```python
from build123d import *

# Parameters (mm, degrees)
SKETCH1_R           = 1.4
BOSS_EXTRUDE1_DEPTH = 2
BOSS_EXTRUDE2_START = -12.5
BOSS_EXTRUDE2_DEPTH = 10
SKETCH2_R           = 2
CUT_EXTRUDE1_DEPTH  = 40.088742751
CUT_EXTRUDE2_START  = -4
SKETCH2_3_R         = 2
CUT_EXTRUDE2_DEPTH  = 36.088742751
SKETCH4_W           = 3.030010437
SKETCH4_H           = 28.00665459
CUT_EXTRUDE3_DEPTH  = 40.088742751


# Read off the part's stored shape, not the designer's step: Boss-Extrude2
with BuildPart() as part:
    # Sketch1 → Boss-Extrude1 (new body)
    with BuildSketch(Plane.XY):
        with BuildLine():
            Line((7.5, -2.5), (7.5, 6.273123532))
            ThreePointArc((7.5, 6.273123532), (6.401650429, 8.924773961), (3.75, 10.023123532))
            Line((3.75, 10.023123532), (0, 10.023123532))
            Line((0, 10.023123532), (0, 13))
            Line((0, 13), (-29.5, 13))
            Line((-29.5, 13), (-29.5, 10.023123532))
            Line((-29.5, 10.023123532), (-33.25, 10.023123532))
            ThreePointArc((-33.25, 10.023123532), (-35.901650429, 8.924773961), (-37, 6.273123532))
            Line((-37, 6.273123532), (-37, -2.5))
            Line((-37, -2.5), (7.5, -2.5))
        make_face()
        with Locations((3.75, 6.273123532)):
            Circle(SKETCH1_R, mode=Mode.SUBTRACT)
        with Locations((-33.25, 6.273123532)):
            Circle(SKETCH1_R, mode=Mode.SUBTRACT)
    extrude(amount=BOSS_EXTRUDE1_DEPTH)

    # Boss-Extrude2 outline → Boss-Extrude2 (add)
    with BuildSketch(Plane(origin=(0, 0, 0), x_dir=(1, 0, 0), z_dir=(0, 1, 0)).offset(BOSS_EXTRUDE2_START)):
        Polygon((7.5, 44.633095244), (-37, 0.133095244), (-37, -2), (7.5, -2), align=None)
    extrude(amount=BOSS_EXTRUDE2_DEPTH)

    # Sketch2 → Cut-Extrude1 (cut, through all)
    with BuildSketch(Plane(origin=(-18.566547622, 0, -18.566547622), x_dir=(-0.7071067811865457, 0, 0.7071067811865495), z_dir=(-0.7071067811865495, 0, -0.7071067811865457))):
        with Locations((4.603838354, -7.5)):
            Circle(SKETCH2_R)
        with Locations((-15.396161646, -7.5)):
            Circle(SKETCH2_R)
    extrude(amount=-CUT_EXTRUDE1_DEPTH, mode=Mode.SUBTRACT)

    # Sketch2<3> → Cut-Extrude2 (cut, through all)
    # profile 1 of 2: a face of its own
    with BuildSketch(Plane(origin=(-18.566547622, 0, -18.566547622), x_dir=(-0.7071067811865457, 0, 0.7071067811865495), z_dir=(-0.7071067811865495, 0, -0.7071067811865457)).offset(CUT_EXTRUDE2_START)):
        Polygon((8.529820185, -7.5), (6.566829269, -4.1), (2.640847439, -4.1), (0.677856524, -7.5), (2.640847439, -10.9), (6.566829269, -10.9), align=None)
        with Locations((4.603838354, -7.5)):
            Circle(SKETCH2_3_R, mode=Mode.SUBTRACT)
    # profile 2 of 2: a face of its own
    with BuildSketch(Plane(origin=(-18.566547622, 0, -18.566547622), x_dir=(-0.7071067811865457, 0, 0.7071067811865495), z_dir=(-0.7071067811865495, 0, -0.7071067811865457)).offset(CUT_EXTRUDE2_START)):
        Polygon((-11.470179815, -7.5), (-13.433170731, -4.1), (-17.359152561, -4.1), (-19.322143476, -7.5), (-17.359152561, -10.9), (-13.433170731, -10.9), align=None)
        with Locations((-15.396161646, -7.5)):
            Circle(SKETCH2_3_R, mode=Mode.SUBTRACT)
    extrude(amount=-CUT_EXTRUDE2_DEPTH, mode=Mode.SUBTRACT)

    # Sketch4 → Cut-Extrude3 (cut, through all)
    with BuildSketch(Plane(origin=(-18.566547622, 0, -18.566547622), x_dir=(-0.7071067811865457, 0, 0.7071067811865495), z_dir=(-0.7071067811865495, 0, -0.7071067811865457))):
        with Locations((27.583843573, 1.503327295)):
            Rectangle(SKETCH4_W, SKETCH4_H)
    extrude(amount=-CUT_EXTRUDE3_DEPTH, mode=Mode.SUBTRACT)


solid = part.part
```
Check sheet for the modelled part. Datum: model origin and axes. Units: mm. A direction names the side the tool comes from. Round coordinates to 2 decimals unless told otherwise and drop trailing zeros. Order: outer loops, then holes, each group sorted by start corner. A loop starts at its lowest first (then second) coordinate and runs counter-clockwise, first axis right, second up. Notation, with made-up numbers: (-25, 14.25) -> (12, 14.25) arc R29 ccw to (12, 52.25) -> close; hole circle Ø10 at (43, 48.5). An arc over 180 degrees is marked (long way). Use CSV: the item, a comma, the result in double quotes.
(1) Cross-section at B-B (x = 4.5). Record the boundary of the cut face in (y, z).
Worked out:
outline,"(-12.5, -41.63) -> (-2.5, -41.63) -> (-2.5, 0) -> (5.09, 0) -> (5.09, 2) -> (-12.5, 2) -> close; (7.46, 0) -> (9.95, 0) -> (9.95, 2) -> (7.46, 2) -> close; hole (-10.9, -20.05) -> (-7.5, -22.83) -> (-4.1, -20.05) -> (-4.1, -14.5) -> (-7.5, -11.72) -> (-10.9, -14.5) -> close"
(2) Cross-section at A-A (y = -6.5). Record the boundary of the cut face in (x, z), and give its area (3 significant figures).
Worked out:
outline,"(-37, -0.13) -> (-23.05, -14.09) -> (-20.22, -11.26) -> (-21.36, -10.11) -> (-9.25, 2) -> (-34.87, 2) -> close; (-20.6, -16.54) -> (-8.9, -28.23) -> (-6.08, -25.4) -> (-7.22, -24.26) -> (7.5, -9.54) -> (7.5, 2) -> (0.22, 2) -> (-16.63, -14.85) -> (-17.77, -13.71) -> close; (-6.46, -30.68) -> (7.5, -44.63) -> (7.5, -19.01) -> (-2.48, -28.99) -> (-3.63, -27.85) -> close"
area,"801 mm²"
(3) Draft check along X on faces 6 (the face through (-6.046, -5.941, -25.43)), 7 (the face through (-10, -12.5, -11)), 8 (the face through (-34.55, 9.79, 0.76)). Enter one of: pulls with the +X half, pulls with the -X half, needs draft (parallel to the pull), parting line crosses it, or undercut.
Worked out:
face 6,"undercut"
face 7,"needs draft"
face 8,"pulls with the -X half"
(4) Depth check by flat-ended pin: pin 1 (2 mm diameter, centred on x = 1.5, y = 9.5, fed in from -Z); pin 2 (11 mm diameter, centred on x = 3, z = -16.5, fed in from +Y); pin 3 (2 mm diameter, centred on y = 12, z = 1.5, fed in from -X). Enter the tip coordinate at first touch or a pass-through.
Worked out:
pin 1,"z = 0"
pin 2,"y = -2.5"
pin 3,"x = -29.5"
(5) Cross-section at C-C (z = -21). Record the boundary of the cut face in (x, y).
Worked out:
outline,"(-16.13, -12.5) -> (7.5, -12.5) -> (7.5, -2.5) -> (-16.13, -2.5) -> close; hole (-4.78, -7.5) -> (-2, -10.9) -> (3.55, -10.9) -> (6.33, -7.5) -> (3.55, -4.1) -> (-2, -4.1) -> close"
(6) Material ranges on line 1 along Y through (x, z) = (-33.25, 0.6); line 2 along Y through (x, z) = (5.5, -15.5); line 3 along Z through (x, y) = (-16, 5), recorded low to high. Write a range as from..to.
Worked out:
line 1,"-12.5..4.87, 7.67..10.02"
line 2,"-12.5..-10.9, -4.1..-2.5"
line 3,"0..2"
(7) Cross-section at D-D (x = -11). Record the boundary of the cut face in (y, z).
Worked out:
outline,"(-12.5, -26.13) -> (-2.5, -26.13) -> (-2.5, 0) -> (13, 0) -> (13, 2) -> (-12.5, 2) -> close; hole (-10.9, -7.27) -> (-7.5, -10.04) -> (-4.1, -7.27) -> (-4.1, -1.71) -> (-7.5, 1.06) -> (-10.9, -1.71) -> close"
(8) Tool access check on faces 1 (the face through (5.085, 6.694, 0.986)), 2 (the face through (-31, 10.023, 1)), 3 (the face through (2, -4.1, -20)), 4 (the face through (2, 10.023, 1)), 5 (the face through (-15, 5, 0)). Record the directions out of +Z, -Z, +X, -X, +Y, -Y that give a thin tool (end or side, any length) a straight path to the whole face; none if there is none.
Worked out:
face 1,"+Z, -Z"
face 2,"+Z, -Z, -X, +Y"
face 3,"none"
face 4,"+Z, -Z, +X, +Y"
face 5,"-Z, +X, -X, +Y"
